from build123d import *

# Parameters (mm, degrees)
F0_R      = 97.5
F0_R_2    = 92.5
F1_DEPTH  = 5
F4_W      = 10
F4_H      = 5
F7_DEPTH  = 27.5
F10_DEPTH = 197.501
F11_R     = 1.25
F12_DEPTH = 5


with BuildPart() as f1:
    # F0 (on Top) → F1 (new body)
    with BuildSketch(Plane.XY):
        Circle(F0_R)
        Circle(F0_R_2, mode=Mode.SUBTRACT)
    extrude(amount=F1_DEPTH)

    # F5: sweep along a path in F2
    with BuildLine(Plane.YZ) as f5_path:
        Line((-95, 2.5), (-100, -27.5))
    # F4 (on plane+point) → F5 (sweep)
    with BuildSketch(Plane.XY.offset(-27.5)):
        with Locations((0, -100)):
            Rectangle(F4_W, F4_H)
    sweep(path=f5_path.line)

    # F6 (on face) → F7 (join)
    with BuildSketch(Plane(origin=(0, 0, 0), x_dir=(1, 0, 0), z_dir=(0, 0, -1))):
        with BuildLine():
            Line((-74.6893332041, -62.6717919444), (-70.8591109885, -59.457853896))
            ThreePointArc((-70.8591109885, -59.457853896), (-80.1073498501, -46.25), (-86.9215674227, -31.6368632576))
            Line((-86.9215674227, -31.6368632576), (-91.6200305266, -33.3469639743))
            ThreePointArc((-91.6200305266, -33.3469639743), (-84.437476869, -48.75), (-74.6893332041, -62.6717919444))
        make_face()
        with BuildLine():
            ThreePointArc((86.9215674227, -31.6368632576), (80.1073498501, -46.25), (70.8591109885, -59.457853896))
            Line((70.8591109885, -59.457853896), (74.6893332041, -62.6717919444))
            ThreePointArc((74.6893332041, -62.6717919444), (84.437476869, -48.75), (91.6200305266, -33.3469639743))
            Line((91.6200305266, -33.3469639743), (86.9215674227, -31.6368632576))
        make_face()
    extrude(amount=F7_DEPTH)

    # F9 (on offset) → F10 (cut, through all)
    with BuildSketch(Plane.YZ.offset(100)):
        Polygon((50, 0), (0, 0), (0, -29.4982548803), (101.8575504422, -29.4982548803), (101.8575504422, 5), (50, 5), align=None)
    extrude(amount=-F10_DEPTH, mode=Mode.SUBTRACT)

    # F11 (on face) → F12 (join)
    with BuildSketch(Plane(origin=(0, 0, 0), x_dir=(1, 0, 0), z_dir=(0, 0, -1))):
        with Locations((82.2597355808, -47.5)):
            Circle(F11_R)
        with Locations((-82.2597355808, -47.5)):
            Circle(F11_R)
    extrude(amount=F12_DEPTH)


solid = f1.part
For this review, take the finished solid that the model builds, in its own axes (mm). Round coordinates to 2 decimals unless told otherwise and drop trailing zeros. Loops run counter-clockwise (first coordinate to the right, second up) from the corner with the lowest first, then second, coordinate; pieces in that order, holes last. Notation, with made-up numbers: (14, 87) - (51, 87) arc R21 cw to (51, 112) - close; hole circle Ø8 at (2.5, 68.25). An arc over 180 degrees is marked (long way). Use one line per item in the form item = value.
1) We need section A-A on y = 0. Write out the cut boundary in (x, z), then the cut area to 3 significant figures.
Solutions:
outline = (-97.5, 0) - (-92.5, 0) - (-92.5, 5) - (-97.5, 5) - close; (92.5, 0) - (97.5, 0) - (97.5, 5) - (92.5, 5) - close
area = 50.0 mm2
2) We need section D-D on x = -48. Write out the cut boundary in (y, z).
Solutions:
outline = (-84.87, 0) - (-79.07, 0) - (-79.07, 5) - (-84.87, 5) - close
3) Mouldability with a two-part tool opening along Y and no side actions: class faces 1 (the face through (81, 50, 3)), 2 (the face through (-5, -98, -13)), 3 (the face through (-2.77, -92.46, 2.46)) as pulls with the +Y half, pulls with the -Y half, needs draft (parallel to the pull), parting line crosses it, or undercut.
Solutions:
face_1 = pulls with the +Y half
face_2 = needs draft
face_3 = undercut
4) Wall thickness on probe 1 along X at (y, z) = (0, 2); probe 2 along Y at (x, z) = (0, 2.65); probe 3 along X at (y, z) = (-35.5, 2): over which ranges is each line inside the solid? List them lowest first.
Solutions:
probe_1 = -97.5 to -92.5, 92.5 to 97.5
probe_2 = -97.5 to -92.5
probe_3 = -90.81 to -85.42, 85.42 to 90.81
5) We need section B-B on z = -2. Write out the cut boundary in (x, y).
Solutions:
outline = circle Ø2.5 at (-82.26, 47.5); (-5, -98.25) - (5, -98.25) - (5, -93.25) - (-5, -93.25) - close; circle Ø2.5 at (82.26, 47.5)
6) Clearance check with flat-ended pins moving along their axes: P1, Ø0.8, axis at x = -82, y = 47, coming from the -Z side; P2, Ø6, axis at y = -20, z = -2.5, coming from the +X side; P3, Ø10, axis at y = -69.5, z = -1, coming from the -X side. State where each tip first meets the part, or that it passes through.
Solutions:
P1 = -5
P2 = 95.76
P3 = -73.03
7) We need section C-C on y = -48. Write out the cut boundary in (x, z), then the cut area to 3 significant figures.
Solutions:
outline = (-84.87, 0) - (-79.07, 0) - (-79.07, 5) - (-84.87, 5) - close; (79.07, 0) - (84.87, 0) - (84.87, 5) - (79.07, 5) - close
area = 57.9 mm2
